Can you work these out from the model? Positions are in its coordinate system, mm. Round coordinates to 2 decimals unless told otherwise and drop trailing zeros. Order: outer loops, then holes, each group sorted by start corner. A loop starts at its lowest first (then second) coordinate and runs counter-clockwise, first axis right, second up. Notation, with made-up numbers: (89.5, 48) -> (116.5, 48) arc R16 cw to (116.5, 56) -> close; hole circle Ø4 at (-31.75, 76.5). An arc over 180 degrees is marked (long way). One line per item, written item: value.
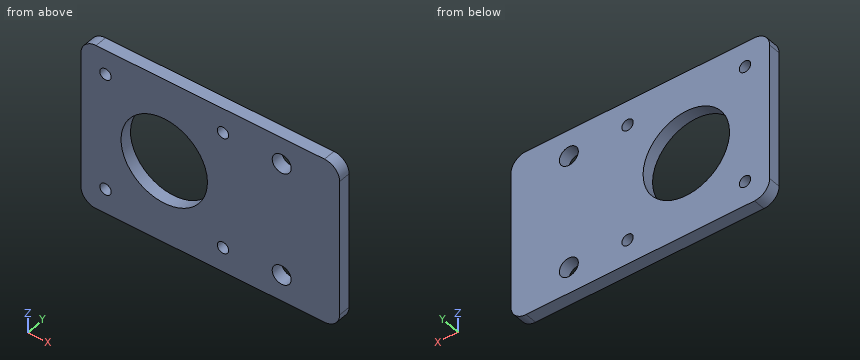
```python
from build123d import *

# Parameters (mm, degrees)
SKETCH1_W           = 68.3
SKETCH1_H           = 44
BOSS_EXTRUDE1_DEPTH = 3.2
SKETCH2_R           = 11.4
SKETCH2_R_2         = 2.5
SKETCH2_R_3         = 1.5
CUT_EXTRUDE2_DEPTH  = 41.748772988
FILLET1_R           = 4


with BuildPart() as part:
    # Sketch1 → Boss-Extrude1 (new body)
    with BuildSketch(Plane(origin=(0, 0, 0), x_dir=(1, 0, 0), z_dir=(0, 1, 0))):
        Rectangle(SKETCH1_W, SKETCH1_H)
    extrude(amount=BOSS_EXTRUDE1_DEPTH)

    # Sketch2 → Cut-Extrude2 (cut, through all)
    with BuildSketch(Plane(origin=(0, 3.2, 0), x_dir=(1, 0, 0), z_dir=(0, 1, 0))):
        with Locations(Location((-12.15, 0, 0), (0, 0, 270))):
            Circle(SKETCH2_R)
        with Locations(Location((18.85, 15, 0), (0, 0, 270))):
            Circle(SKETCH2_R_2)
        with Locations(Location((18.85, -15, 0), (0, 0, 270))):
            Circle(SKETCH2_R_2)
        with Locations(Location((-27.65, 15.5, 0), (0, 0, 270))):
            Circle(SKETCH2_R_3)
        with Locations(Location((3.35, 15.5, 0), (0, 0, 270))):
            Circle(SKETCH2_R_3)
        with Locations(Location((3.35, -15.5, 0), (0, 0, 270))):
            Circle(SKETCH2_R_3)
        with Locations(Location((-27.65, -15.5, 0), (0, 0, 270))):
            Circle(SKETCH2_R_3)
    extrude(amount=-CUT_EXTRUDE2_DEPTH, mode=Mode.SUBTRACT)

    # Fillet1
    fillet1_edges = [part.edges().sort_by_distance(p)[0] for p in [
        (34.15, 1.6, 22),
        (-34.15, 1.6, 22),
        (-34.15, 1.6, -22),
        (34.15, 1.6, -22),
    ]]
    fillet(fillet1_edges, radius=FILLET1_R)


solid = part.part
```
Q1. Please list where these lines run through material, in increasing order: line 1 along X through (y, z) = (2, 15.5); line 2 along Z through (x, y) = (20.5, 2.8); line 3 along X through (y, z) = (2.4, 0.5).
Answers below:
line 1: -34.15 to -29.15, -26.15 to 1.85, 4.85 to 16.4, 21.3 to 34.15
line 2: -22 to -16.88, -13.12 to 13.12, 16.88 to 22
line 3: -34.15 to -23.54, -0.76 to 34.15
Q2. I want a section at D-D on z = -0.5. List the corners of the cut face in (x, y) for me, plus the area to 3 significant figures.
Answers below:
outline: (-34.15, 0) -> (-23.54, 0) -> (-23.54, 3.2) -> (-34.15, 3.2) -> close; (-0.76, 0) -> (34.15, 0) -> (34.15, 3.2) -> (-0.76, 3.2) -> close
area: 146 mm^2
Q3. I want a section at B-B on x = -12.15. List the corners of the cut face in (y, z) for me.
Answers below:
outline: (0, -22) -> (3.2, -22) -> (3.2, -11.4) -> (0, -11.4) -> close; (0, 11.4) -> (3.2, 11.4) -> (3.2, 22) -> (0, 22) -> close
Q4. I want a section at A-A on x = 18.85. List the corners of the cut face in (y, z) for me.
Answers below:
outline: (0, -22) -> (3.2, -22) -> (3.2, -17.5) -> (0, -17.5) -> close; (0, -12.5) -> (3.2, -12.5) -> (3.2, 12.5) -> (0, 12.5) -> close; (0, 17.5) -> (3.2, 17.5) -> (3.2, 22) -> (0, 22) -> close
Q5. Will this pin go through, and if not, where does the flat tip stop? pin 1 Ø2.5 at (x, z) = (3.35, -15.5) entering from +Y.
Answers below:
pin 1: through
Q6. I want a section at C-C on y = 2.1. List the corners of the cut face in (x, z) for me.
Answers below:
outline: (-34.15, -18) arc R4 ccw to (-30.15, -22) -> (30.15, -22) arc R4 ccw to (34.15, -18) -> (34.15, 18) arc R4 ccw to (30.15, 22) -> (-30.15, 22) arc R4 ccw to (-34.15, 18) -> close; hole circle Ø3 at (-27.65, -15.5); hole circle Ø3 at (-27.65, 15.5); hole circle Ø22.8 at (-12.15, 0); hole circle Ø3 at (3.35, -15.5); hole circle Ø3 at (3.35, 15.5); hole circle Ø5 at (18.85, -15); hole circle Ø5 at (18.85, 15)
